The figure shows three views and two pictorial views of one solid part (mm, origin at its lowest corner). Answer the questions. A direction names the side the tool comes from. Round coordinates to 2 decimals unless told otherwise and drop trailing zeros. Order: outer loops, then holes, each group sorted by start corner. A loop starts at its lowest first (then second) coordinate and runs counter-clockwise, first axis right, second up. Notation, with made-up numbers: (-1.75, 20.25) -> (22.25, 20.25) arc R29 cw to (22.25, 59.25) -> close; hole circle Ø1 at (16.25, 15). An arc over 180 degrees is marked (long way). Return JSON: item names as keys, results as strings. Group by question number.
(1) The part is cut by section C-C (y = 30). Determine the outline of the cut face in (x, z), plus the area to 3 significant figures.
(2) The part is cut by section B-B (x = 14). Determine the outline of the cut face in (y, z), plus the area to 3 significant figures.
(3) The part is cut by section A-A (z = 20.5). Determine the outline of the cut face in (x, y), plus the area to 3 significant figures.
(4) Determine the mould class of the marked faces 1, 2 and 3 for opening direction Z: +Z half, -Z half, draft (parallel to the pull), parting line (faces both ways), or undercut.
(5) Consider line 1 (Z direction, x = 31, y = 22.5); line 2 (Z direction, x = 10, y = 1.1); line 3 (X direction, y = 36, z = 13.5). Determine where each line is inside the solid, lowest interval first. Write a range as [from, to].
(6) Which of the six approach directions +Z, -Z, +X, -X, +Y, -Y give full straight-line access (tool end or side, diameter ignored) to the marked faces 4 and 5?
(7) The part is cut by section D-D (x = 25). Determine the outline of the cut face in (y, z), plus the area to 3 significant figures.
(8) Each of these flat-tipped pins is pushed along its axis until it touches: pin 1 (5 mm diameter, centred on x = 23.5, z = 16, fed in from +Y); pin 2 (9 mm diameter, centred on x = 10, z = 17.5, fed in from +Y); pin 3 (15 mm diameter, centred on y = 20, z = 18.5, fed in from -X). Where does it stop, or does it pass through?
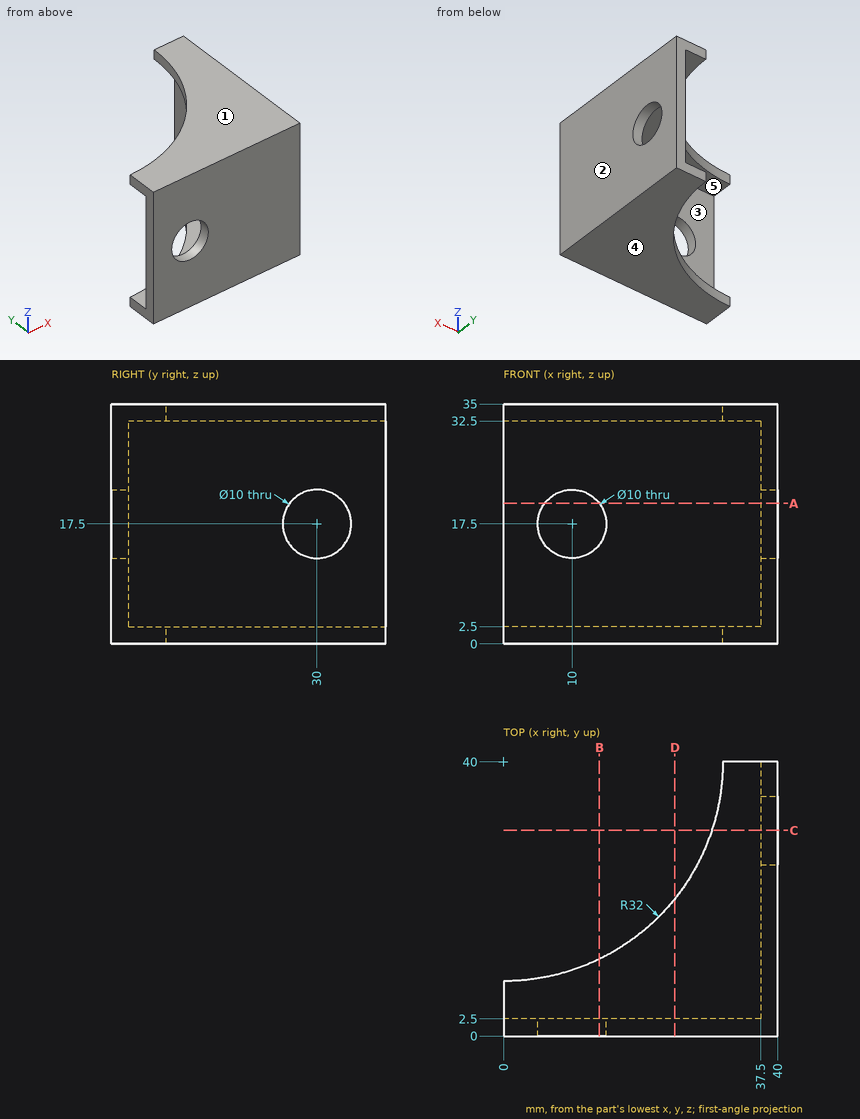
Answer below:
{
 "1": {"outline": "(30.4, 0) -> (40, 0) -> (40, 12.5) -> (37.5, 12.5) -> (37.5, 2.5) -> (30.4, 2.5) -> close; (30.4, 32.5) -> (37.5, 32.5) -> (37.5, 22.5) -> (40, 22.5) -> (40, 35) -> (30.4, 35) -> close", "area": "98.0 mm²"},
 "2": {"outline": "(0, 0) -> (11.23, 0) -> (11.23, 2.5) -> (2.5, 2.5) -> (2.5, 14.5) -> (0, 14.5) -> close; (0, 20.5) -> (2.5, 20.5) -> (2.5, 32.5) -> (11.23, 32.5) -> (11.23, 35) -> (0, 35) -> close", "area": "116 mm²"},
 "3": {"outline": "(0, 0) -> (6, 0) -> (6, 2.5) -> (0, 2.5) -> close; (14, 0) -> (40, 0) -> (40, 26) -> (37.5, 26) -> (37.5, 2.5) -> (14, 2.5) -> close; (37.5, 34) -> (40, 34) -> (40, 40) -> (37.5, 40) -> close", "area": "154 mm²"},
 "4": {"face 1": "+Z half", "face 2": "draft", "face 3": "undercut"},
 "5": {"line 1": "z = [0, 2.5], [32.5, 35]", "line 2": "z = [0, 12.5], [22.5, 35]", "line 3": "x = [37.5, 40]"},
 "6": {"face 4": "-Z, +X, -X, +Y, -Y", "face 5": "-X, +Y"},
 "7": {"outline": "(0, 0) -> (20.03, 0) -> (20.03, 2.5) -> (2.5, 2.5) -> (2.5, 32.5) -> (20.03, 32.5) -> (20.03, 35) -> (0, 35) -> close", "area": "175 mm²"},
 "8": {"pin 1": "stops at y = 2.5", "pin 2": "passes through", "pin 3": "stops at x = 37.5"}
}
